The listing builds one solid part. Answer for the finished solid, in the listing's coordinates (mm). Face numbers are marked on the shaded views. Coordinates: 2 decimals unless noted, no trailing zeros. Order: outer loops, then holes, each group sorted by start corner. A loop starts at its lowest first (then second) coordinate and runs counter-clockwise, first axis right, second up. Notation, with made-up numbers: (33, 71) - (51, 71) arc R29 cw to (51, 95) - close; hole circle Ø3 at (54.25, -33). An arc over 180 degrees is marked (long way). Use one line per item in the form item = value. Start each with the question number.
Item 1: Consider line 1 along Z through (x, y) = (-2.5, -2.1); line 2 along Z through (x, y) = (-0.5, -0.55); line 3 along X through (y, z) = (-1.75, 1.25). Determine where each line is inside the solid, lowest interval first. Write a range as [from, to].
Item 2: The mould has two halves that part along X. Classify the marked faces 1, 2 and 3: released by +X, released by -X, zero draft, split by the parting line, or undercut.
Item 3: This flat-tipped pin is pushed along its axis until it touches: pin 1 Ø1.5 at (x, y) = (-1.5, -2) entering from +Z. Where does it stop, or does it pass through?
Item 4: Section C-C, the plane y = -1.9 is taken. Write down the section's boundary in (x, z), and give its area (3 significant figures).
Item 5: Section D-D, the plane y = -0.5 is taken. Write down the section's boundary in (x, z), and give its area (3 significant figures).
from build123d import *

# Parameters (mm, degrees)
F0_R     = 4.95
F0_R_2   = 3.85
F0_R_3   = 2
F1_DEPTH = 2.5
F2_DEPTH = 3.19
F3_SIZE2 = 2.49999
F3_SIZE  = 2.49999


# Not quite as in the source:
# - a fillet or chamfer is up to 0.001 mm smaller than in the source, because OpenCascade refuses the exact size


with BuildPart() as f1:
    # F0 (on Front) → F1 (new body)
    with BuildSketch(Plane.XZ):
        Circle(F0_R)
        Circle(F0_R_2, mode=Mode.SUBTRACT)
        Circle(F0_R_2)
        Circle(F0_R_3, mode=Mode.SUBTRACT)
        Circle(F0_R_3)
    extrude(amount=F1_DEPTH)

    # F0 (on Front) → F2 (cut)
    with BuildSketch(Plane.XZ):
        Circle(F0_R_3)
    extrude(amount=F2_DEPTH, mode=Mode.SUBTRACT)

    # F3 (size 2.5 and 2.5 in the source; OpenCascade refuses exactly that, so slightly less here)
    f3_edges = [f1.edges().sort_by_distance(p)[0] for p in [
        (-2, -2.5, 0),
    ]]
    chamfer(f3_edges, length=F3_SIZE, length2=F3_SIZE2)


solid = f1.part
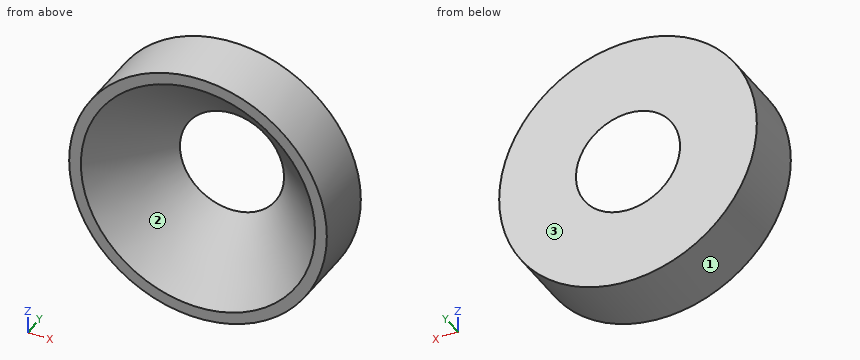
Response:
q1.line_1 = [-4.27, -3.25], [3.25, 4.27]
q1.line_2 = [-4.92, -2.5], [2.5, 4.92]
q1.line_3 = [-4.79, -3.54], [3.54, 4.79]
q2.face_1 = split by the parting line
q2.face_2 = undercut
q2.face_3 = zero draft
q3.pin_1 = 4.89
q4.outline = circle Ø9.9 at (0, 0); hole circle Ø7.8 at (0, 0)
q4.area = 29.2 mm2
q5.outline = circle Ø9.9 at (0, 0); hole circle Ø5 at (0, 0)
q5.area = 57.3 mm2
